Read the model definition and answer for the solid it produces. Units are mm, in the model's axes. Coordinates: 2 decimals unless noted, no trailing zeros. Order: outer loops, then holes, each group sorted by start corner. A loop starts at its lowest first (then second) coordinate and runs counter-clockwise, first axis right, second up. Notation, with made-up numbers: (49.5, -9) -> (68.5, -9) arc R15 ccw to (68.5, 4) -> close; hole circle Ø1 at (53.5, -18). An arc over 180 degrees is marked (long way). Answer as a JSON object with one key per item and string values. Group by question number.
1) Section B-B on x = 8 is taken. Determine the outline of the cut face in (y, z), and give its area (3 significant figures).
2) Given pin 1 (6 mm diameter, centred on y = -18.5, z = -17, fed in from -X); pin 2 (5 mm diameter, centred on x = -12.5, y = -4.5, fed in from +Z); pin 3 (8 mm diameter, centred on y = -14.5, z = -19.5, fed in from -X), each flat-ended and moving along its own axis, determine where each tip first touches the part or whether it passes through.
3) Section A-A on x = 0 is taken. Determine the outline of the cut face in (y, z), and give its area (3 significant figures).
4) Consider L1, parallel to Z at x = 0, y = -18.5; L2, parallel to Z at x = 1, y = -6.75; L3, parallel to X at y = -12, z = -29. Determine where each line is inside the solid, lowest interval first.
from build123d import *

# Parameters (mm, degrees)
F1_DEPTH = 25
F2_R     = 1.5875
F3_DEPTH = 25


with BuildPart() as f1:
    # F0 (on Front) → F1 (new body)
    with BuildSketch(Plane.XZ):
        with BuildLine():
            Line((-17.3205080757, 10), (0, 0))
            Line((0, 0), (17.3205080757, 10))
            ThreePointArc((17.3205080757, 10), (0, 20), (-17.3205080757, 10))
        make_face()
        with BuildLine():
            ThreePointArc((19.0525588833, 11), (0, 22), (-19.0525588833, 11))
            Line((-19.0525588833, 11), (-17.3205080757, 10))
            ThreePointArc((-17.3205080757, 10), (0, 20), (17.3205080757, 10))
            Line((17.3205080757, 10), (19.0525588833, 11))
        make_face()
        with BuildLine():
            Line((19.3185165258, 5.1763809021), (21.2503681784, 5.6940189923))
            ThreePointArc((21.2503681784, 5.6940189923), (20.3253497152, 8.419035512), (19.0525588833, 11))
            Line((19.0525588833, 11), (17.3205080757, 10))
            ThreePointArc((17.3205080757, 10), (18.4775906502, 7.6536686473), (19.3185165258, 5.1763809021))
        make_face()
        with BuildLine():
            Line((17.3205080757, 10), (0, 0))
            Line((0, 0), (19.3185165258, 5.1763809021))
            ThreePointArc((19.3185165258, 5.1763809021), (18.4775906502, 7.6536686473), (17.3205080757, 10))
        make_face()
        with BuildLine():
            Line((0, 0), (19.3185165258, -5.1763809021))
            ThreePointArc((19.3185165258, -5.1763809021), (19.8288972275, -2.6105238444), (20, 0))
            ThreePointArc((20, 0), (19.8288972275, 2.6105238444), (19.3185165258, 5.1763809021))
            Line((19.3185165258, 5.1763809021), (0, 0))
        make_face()
        with BuildLine():
            add(Edge.make_bspline(
                [(19.3185165258, -5.1763809021), (21.3890688866, 2.5510257083), (22.0268253137, 2.7962415134), (21.2503681784, 5.6940189923)],
                knots=[0, 0, 0, 0, 11.0407266369, 11.0407266369, 11.0407266369, 11.0407266369], degree=3))
            Line((21.2503681784, 5.6940189923), (19.3185165258, 5.1763809021))
            ThreePointArc((19.3185165258, 5.1763809021), (19.8288972275, 2.6105238444), (20, 0))
            ThreePointArc((20, 0), (19.8288972275, -2.6105238444), (19.3185165258, -5.1763809021))
        make_face()
        with BuildLine():
            Line((0, 0), (17.3205080757, -10))
            ThreePointArc((17.3205080757, -10), (18.4775906502, -7.6536686473), (19.3185165258, -5.1763809021))
            Line((19.3185165258, -5.1763809021), (0, 0))
        make_face()
        with BuildLine():
            ThreePointArc((-17.3205080757, -10), (0, -20), (17.3205080757, -10))
            Line((17.3205080757, -10), (0, 0))
            Line((0, 0), (-17.3205080757, 10))
            ThreePointArc((-17.3205080757, 10), (-19.8288972275, 2.6105238444), (-19.3185165258, -5.1763809021))
            ThreePointArc((-19.3185165258, -5.1763809021), (-18.4775906502, -7.6536686473), (-17.3205080757, -10))
        make_face()
        with BuildLine():
            Line((-10, -40), (10, -40))
            add(Edge.make_bspline(
                [(13.6086616321, -17.2859575547), (11.1605636245, -23.1152490417), (10, -29.3919833148), (10, -40)],
                knots=[9.0417028431, 9.0417028431, 9.0417028431, 9.0417028431, 30.8802499745, 30.8802499745, 30.8802499745, 30.8802499745], degree=3))
            ThreePointArc((13.6086616321, -17.2859575547), (13.1773214563, -17.6169860997), (12.7379323807, -17.9372539332))
            ThreePointArc((12.7379323807, -17.9372539332), (-0.543681065, -21.9932810399), (-13.6086616321, -17.2859575547))
            add(Edge.make_bspline(
                [(-13.6086616321, -17.2859575547), (-11.1605636245, -23.1152490417), (-10, -29.3919833148), (-10, -40)],
                knots=[9.0417028431, 9.0417028431, 9.0417028431, 9.0417028431, 30.8802499745, 30.8802499745, 30.8802499745, 30.8802499745], degree=3))
        make_face()
        with BuildLine():
            add(Edge.make_bspline(
                [(-17.3205080757, -10), (-15.8565136374, -12.5357127491), (-14.6222352267, -14.8724855827), (-13.6086616321, -17.2859575547)],
                knots=[0, 0, 0, 0, 9.0417028431, 9.0417028431, 9.0417028431, 9.0417028431], degree=3))
            ThreePointArc((-13.6086616321, -17.2859575547), (-0.543681065, -21.9932810399), (12.7379323807, -17.9372539332))
            Line((12.7379323807, -17.9372539332), (17.3205080757, -10))
            ThreePointArc((17.3205080757, -10), (0, -20), (-17.3205080757, -10))
        make_face()
        with BuildLine():
            ThreePointArc((-19.0525588833, 11), (-20.3253497152, 8.419035512), (-21.2503681784, 5.6940189923))
            add(Edge.make_bspline(
                [(-19.3185165258, -5.1763809021), (-21.3890688866, 2.5510257083), (-22.0268253137, 2.7962415134), (-21.2503681784, 5.6940189923)],
                knots=[0, 0, 0, 0, 11.0407266369, 11.0407266369, 11.0407266369, 11.0407266369], degree=3))
            ThreePointArc((-19.3185165258, -5.1763809021), (-19.8288972275, 2.6105238444), (-17.3205080757, 10))
            Line((-17.3205080757, 10), (-19.0525588833, 11))
        make_face()
        with BuildLine():
            ThreePointArc((12.7379323807, -17.9372539332), (13.1773214563, -17.6169860997), (13.6086616321, -17.2859575547))
            add(Edge.make_bspline(
                [(17.3205080757, -10), (15.8565136374, -12.5357127491), (14.6222352267, -14.8724855827), (13.6086616321, -17.2859575547)],
                knots=[0, 0, 0, 0, 9.0417028431, 9.0417028431, 9.0417028431, 9.0417028431], degree=3))
            Line((17.3205080757, -10), (12.7379323807, -17.9372539332))
        make_face()
    extrude(amount=F1_DEPTH)

    # F2 (on face) → F3 (cut)
    with BuildSketch(Plane.XZ.offset(25)):
        Circle(F2_R)
    extrude(amount=-F3_DEPTH, mode=Mode.SUBTRACT)


solid = f1.part
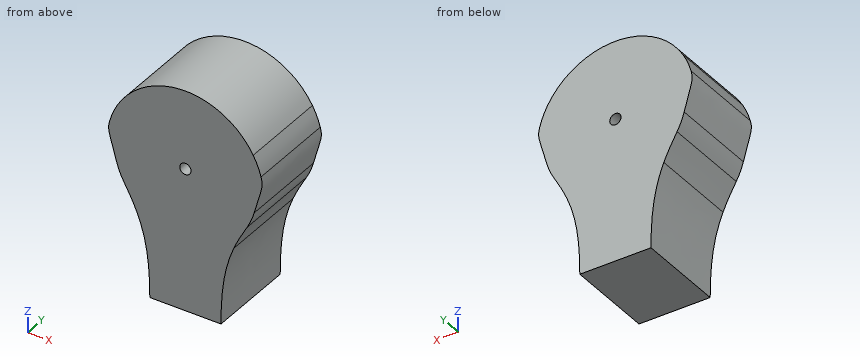
Worked answers:
{
 "1": {"outline": "(-25, -40) -> (0, -40) -> (0, 20.49) -> (-25, 20.49) -> close", "area": "1,510 mm²"},
 "2": {"pin 1": "stops at x = -15.14", "pin 2": "stops at z = 19.6", "pin 3": "stops at x = -14.4"},
 "3": {"outline": "(-25, -40) -> (0, -40) -> (0, -1.59) -> (-25, -1.59) -> close; (-25, 1.59) -> (0, 1.59) -> (0, 22) -> (-25, 22) -> close", "area": "1,470 mm²"},
 "4": {"L1": "z = -40 to -1.59, 1.59 to 22", "L2": "z = -40 to -1.23, 1.23 to 21.98", "L3": "x = -10.58 to 10.58"}
}
